from build123d import *

# Parameters (mm, degrees)
SKETCH2_W           = 76.2
SKETCH2_H           = 114.3
BOSS_EXTRUDE1_DEPTH = 12.7
SKETCH4_W           = 12.7
SKETCH4_H           = 3.81
CUT_EXTRUDE1_DEPTH  = 76.2
SKETCH5_W           = 12.7
SKETCH5_H           = 3.81
CUT_EXTRUDE2_DEPTH  = 76.2


with BuildPart() as part:
    # Sketch2 → Boss-Extrude1 (new body)
    with BuildSketch(Plane(origin=(0, 0, 0), x_dir=(1, 0, 0), z_dir=(0, 1, 0))):
        Rectangle(SKETCH2_W, SKETCH2_H)
    extrude(amount=BOSS_EXTRUDE1_DEPTH)

    # Sketch4 → Cut-Extrude1 (cut)
    with BuildSketch(Plane(origin=(38.1, 0, 0), x_dir=(0, 0, -1), z_dir=(1, 0, 0))):
        with Locations((-38.1, 10.795)):
            Rectangle(SKETCH4_W, SKETCH4_H)
    cut_extrude1 = extrude(amount=-CUT_EXTRUDE1_DEPTH, mode=Mode.SUBTRACT)

    # Mirror1: Cut-Extrude1 across plane
    add(cut_extrude1.mirror(Plane.XY), mode=Mode.SUBTRACT)

    # Sketch5 → Cut-Extrude2 (cut)
    with BuildSketch(Plane(origin=(38.1, 0, 0), x_dir=(0, 0, -1), z_dir=(1, 0, 0))):
        with Locations((0, 10.795)):
            Rectangle(SKETCH5_W, SKETCH5_H)
    extrude(amount=-CUT_EXTRUDE2_DEPTH, mode=Mode.SUBTRACT)


solid = part.part
Source: CAD feature listing. Evaluate the final solid. Frame: model axes, mm. A direction names the side the tool comes from. Coordinates: 2 decimals unless noted, no trailing zeros. Write each loop counter-clockwise with the first axis right and the second up, starting at its lowest first coordinate (ties: lowest second). Pieces come first, ordered by that corner, then holes. Notation, with made-up numbers: M 7.25,-30 L 27.25,-30 A33 ccw 27.25,1 Z; hole C -1,-36.5 d2. An arc over 180 degrees is marked long. Use a Markdown table: item, result.
1) Section B-B, the plane z = -37.5. Output: boundary loops of the cut face in (x, y), then the cut area to 3 significant figures.
Conclusion:
| item | result |
|---|---|
| outline | M -38.1,0 L 38.1,0 L 38.1,8.89 L -38.1,8.89 Z |
| area | 677 mm^2 |
2) First-contact query: pin 1 Ø4 at (x, z) = (16, 37.5) entering from +Y. Flat tip, straight axial feed; report the tip coordinate or a pass-through.
Conclusion:
| item | result |
|---|---|
| pin 1 | stops at y = 8.89 |
3) Section A-A, the plane x = -31. Output: boundary loops of the cut face in (y, z), then the cut area to 3 significant figures.
Conclusion:
| item | result |
|---|---|
| outline | M 0,-57.15 L 12.7,-57.15 L 12.7,-44.45 L 8.89,-44.45 L 8.89,-31.75 L 12.7,-31.75 L 12.7,-6.35 L 8.89,-6.35 L 8.89,6.35 L 12.7,6.35 L 12.7,31.75 L 8.89,31.75 L 8.89,44.45 L 12.7,44.45 L 12.7,57.15 L 0,57.15 Z |
| area | 1,310 mm^2 |
4) Ray query, L1, parallel to Z at x = 27.5, y = 11.25; L2, parallel to Y at x = -28.5, z = -32. Return the intervals inside material, ascending.
Conclusion:
| item | result |
|---|---|
| L1 | z = -57.15 to -44.45, -31.75 to -6.35, 6.35 to 31.75, 44.45 to 57.15 |
| L2 | y = 0 to 8.89 |
5) Mould query, pull axis Z, two halves, no side actions, for faces 3 (the flat face through (-1, 12.7, -51)), 4 (the flat face through (-1, 6, 57.15)), 5 (the flat face through (1, 11, 6.35)), 6 (the flat face through (-1, 6, -57.15)). Classes: pulls with the +Z half, pulls with the -Z half, needs draft (parallel to the pull), parting line crosses it, or undercut.
Conclusion:
| item | result |
|---|---|
| face 3 | needs draft |
| face 4 | pulls with the +Z half |
| face 5 | undercut |
| face 6 | pulls with the -Z half |
6) Reachability of faces 1 (the flat face through (1, 11, 44.45)), 2 (the flat face through (-1, 12.7, 51)) from +Z, -Z, +X, -X, +Y, -Y: full face, straight path, thin tool, end or side. Return the list, or none.
Conclusion:
| item | result |
|---|---|
| face 1 | +X, -X, +Y |
| face 2 | +Z, -Z, +X, -X, +Y |
